```python
from build123d import *

# Parameters (mm, degrees)
BOSS_EXTRUDE1_DEPTH = 31.75
BOSS_EXTRUDE2_DEPTH = 3.81


with BuildPart() as part:
    # Sketch2 → Boss-Extrude1 (new body)
    with BuildSketch(Plane.XY):
        Polygon((2.566321947, 4.445), (3.446203757, 5.969), (-3.446203757, 5.969), (-6.892407514, 0), (-3.446203757, -5.969), (3.446203757, -5.969), (6.892407514, 0), (5.132643893, 0), (2.566321947, -4.445), (-2.566321947, -4.445), (-5.132643893, 0), (-2.566321947, 4.445), align=None)
    extrude(amount=BOSS_EXTRUDE1_DEPTH)

    # Sketch3 → Boss-Extrude2 (add)
    with BuildSketch(Plane(origin=(0, 0, 0), x_dir=(-1, 0, 0), z_dir=(0, 0, -1))):
        with BuildLine():
            Line((-5.132643893, 0), (-3.068091577, -0.816969447))
            ThreePointArc((-3.068091577, -0.816969447), (2.749630657, -1.5875), (-0.826529493, 3.06552997))
            Line((-0.826529493, 3.06552997), (-2.566321947, 4.445))
            Line((-2.566321947, 4.445), (2.566321947, 4.445))
            Line((2.566321947, 4.445), (5.132643893, 0))
            Line((5.132643893, 0), (2.566321947, -4.445))
            Line((2.566321947, -4.445), (-2.566321947, -4.445))
            Line((-2.566321947, -4.445), (-5.132643893, 0))
        make_face()
    extrude(amount=-BOSS_EXTRUDE2_DEPTH)


solid = part.part
```
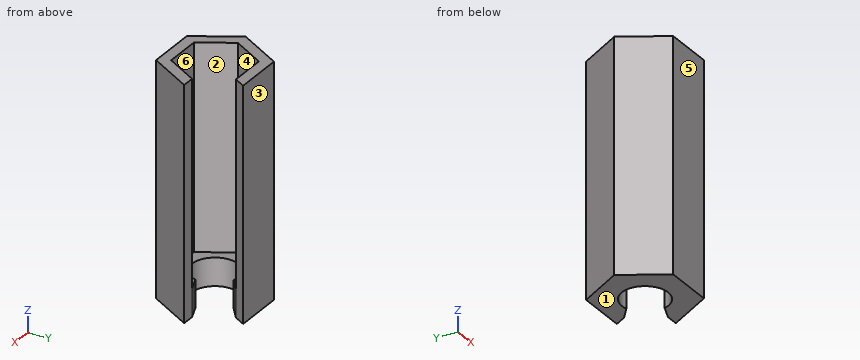
Verification items for the finished model (mm, model axes). Face numbers are marked on the shaded views. A direction names the side the tool comes from. Round coordinates to 2 decimals unless told otherwise and drop trailing zeros. Order: outer loops, then holes, each group sorted by start corner. A loop starts at its lowest first (then second) coordinate and runs counter-clockwise, first axis right, second up. Notation, with made-up numbers: (16.25, 11) - (59.25, 11) arc R28 cw to (59.25, 48) - close; hole circle Ø4 at (37, 77.25). An arc over 180 degrees is marked (long way). Use CSV: the item, a comma, the result in double quotes. Start each with the question number.
1) Thickness scan on L1, parallel to Y at x = -0.75, z = 29.5 (3 decimals); L2, parallel to Y at x = 0, z = 1.15 (3 decimals); L3, parallel to Z at x = -2, y = -3.25. Record the ranges inside material, lowest first.
2) Section check C-C, the plane y = 2.5. Record the cut outline in (x, z).
3) Go/stop test with flat-tipped pins: P1, Ø3, axis at y = 2.5, z = 21.5, coming from the +X side; P2, Ø0.9, axis at x = 6.5, z = 14, coming from the +Y side; P3, Ø3, axis at y = 3.5, z = 13, coming from the +X side. Record where each tip stops, or that it passes through.
4) Section check A-A, the plane x = 0. Record the cut outline in (y, z) (3 decimals), plus the area to 3 significant figures.
5) Section check B-B, the plane z = 21.5. Record the cut outline in (x, y) (3 decimals).
6) Mould release check, pull along Y, two halves, no side actions. Record for the marked faces 3, 4, 5 and 6: +Y half, -Y half, draft (parallel to the pull), parting line (faces both ways), or undercut.
7) Access from +Z, -Z, +X, -X, +Y, -Y to the whole of each face (thin tool, end or side, straight path). Record for the marked faces 1 and 2.
8) Section check D-D, the plane x = 4.5. Record the cut outline in (y, z).
Answers:
1,L1,"y = -5.969 to -4.445, 4.445 to 5.969"
1,L2,"y = -5.969 to -3.175, 3.175 to 5.969"
1,L3,"z = 0 to 3.81"
2,outline,"(-5.45, 0) - (-1.96, 0) - (-1.96, 3.81) - (-3.69, 3.81) - (-3.69, 31.75) - (-5.45, 31.75) - close"
3,P1,"stops at x = -2.82"
3,P2,"stops at y = 0"
3,P3,"stops at x = 2.89"
4,outline,"(-5.969, 0) - (-3.175, 0) - (-3.175, 3.81) - (-4.445, 3.81) - (-4.445, 31.75) - (-5.969, 31.75) - close; (3.175, 0) - (5.969, 0) - (5.969, 31.75) - (4.445, 31.75) - (4.445, 3.81) - (3.175, 3.81) - close"
4,area,"106 mm²"
5,outline,"(-6.892, 0) - (-3.446, -5.969) - (3.446, -5.969) - (6.892, 0) - (5.133, 0) - (2.566, -4.445) - (-2.566, -4.445) - (-5.133, 0) - (-2.566, 4.445) - (2.566, 4.445) - (3.446, 5.969) - (-3.446, 5.969) - close"
6,face 3,"+Y half"
6,face 4,"undercut"
6,face 5,"-Y half"
6,face 6,"undercut"
7,face 1,"-Z, +X, -X, +Y, -Y"
7,face 2,"+Z"
8,outline,"(-4.14, 0) - (-0.25, 0) - (-0.25, 3.81) - (-1.1, 3.81) - (-1.1, 31.75) - (-4.14, 31.75) - close"
